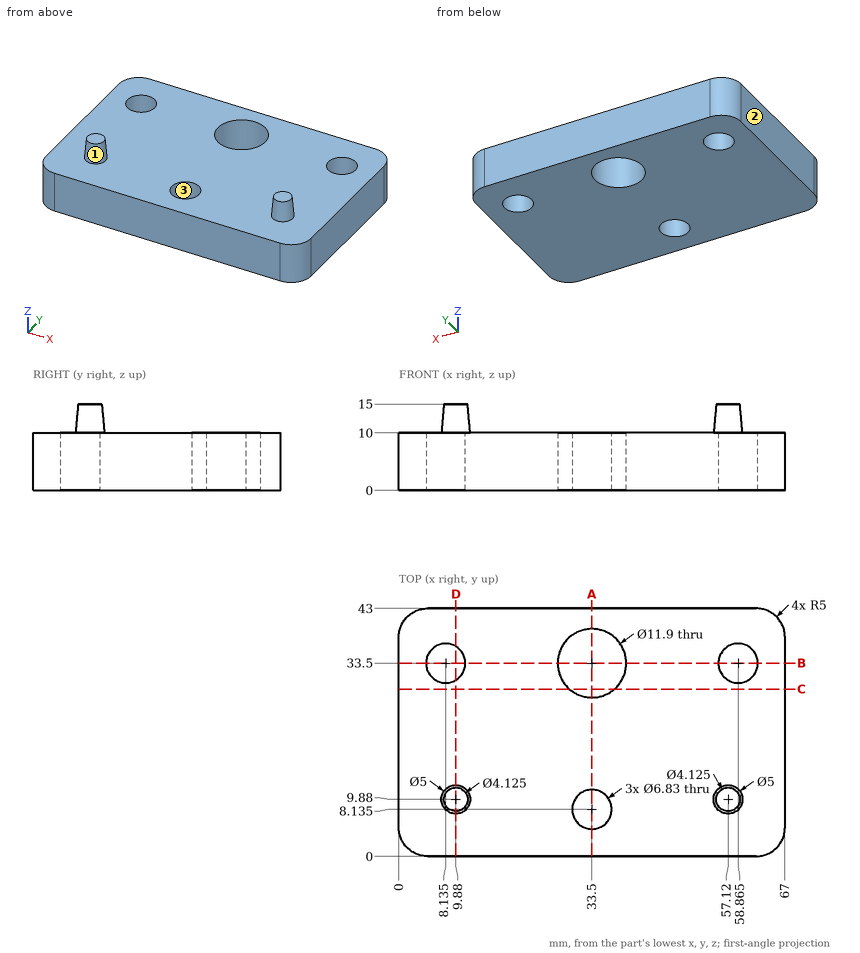
Geometry: see drawing. Coordinates: mm, zero at the bounding-box minimum. Round coordinates to 2 decimals unless told otherwise and drop trailing zeros. Loops run counter-clockwise (first coordinate to the right, second up) from the corner with the lowest first, then second, coordinate; pieces in that order, holes last. Notation, with made-up numbers: M -25,3.5 L -4,3.5 A5 ccw -4,11.5 Z; hole C 25.5,51.25 d7. An arc over 180 degrees is marked long. Use a Markdown table: item, result. Add a question column.
1. Section query A-A on x = 33.5. Return the cut outline in (y, z).
2. Contact query for a flat-ended pin moving along its axis: P1, Ø1.5, axis at x = 15.5, y = 5.5, coming from the +Z side. Output: stop coordinate, or through.
3. Section query D-D on x = 9.88. Return the cut outline in (y, z).
4. Section query B-B on y = 33.5. Return the cut outline in (x, z).
5. Section query C-C on y = 29. Return the cut outline in (x, z).
6. Mould query, pull axis Y, two halves, no side actions, for the marked faces 1, 2 and 3. Classes: pulls with the +Y half, pulls with the -Y half, needs draft (parallel to the pull), parting line crosses it, or undercut.
7. Line query: line 1 (Y direction, x = 33.5, z = 7.5); line 2 (Y direction, x = 35.5, z = 9); line 3 (Z direction, x = 50.5, y = 34.5). Output: solid intervals per line, ascending.
Reported:
| question | item | result |
|---|---|---|
| 1 | outline | M 0,0 L 4.72,0 L 4.72,10 L 0,10 Z; M 11.55,0 L 27.55,0 L 27.55,10 L 11.55,10 Z; M 39.45,0 L 43,0 L 43,10 L 39.45,10 Z |
| 2 | P1 | stops at z = 10 |
| 3 | outline | M 0,0 L 30.56,0 L 30.56,10 L 12.38,10 L 11.94,15 L 7.82,15 L 7.38,10 L 0,10 Z; M 36.44,0 L 43,0 L 43,10 L 36.44,10 Z |
| 4 | outline | M 0,0 L 4.72,0 L 4.72,10 L 0,10 Z; M 11.55,0 L 27.55,0 L 27.55,10 L 11.55,10 Z; M 39.45,0 L 55.45,0 L 55.45,10 L 39.45,10 Z; M 62.28,0 L 67,0 L 67,10 L 62.28,10 Z |
| 5 | outline | M 0,0 L 29.61,0 L 29.61,10 L 0,10 Z; M 37.39,0 L 67,0 L 67,10 L 37.39,10 Z |
| 6 | face 1 | parting line crosses it |
| 6 | face 2 | needs draft |
| 6 | face 3 | undercut |
| 7 | line 1 | y = 0 to 4.72, 11.55 to 27.55, 39.45 to 43 |
| 7 | line 2 | y = 0 to 5.37, 10.9 to 27.9, 39.1 to 43 |
| 7 | line 3 | z = 0 to 10 |
